```python
from build123d import *

# Parameters (mm, degrees)
F0_R     = 3.75
F0_R_2   = 1.75
F1_DEPTH = 3.8
F3_DEPTH = 2.5
F4_DEPTH = 1.2


with BuildPart() as f1:
    # F0 (on Top) → F1 (new body)
    with BuildSketch(Plane.XY):
        with Locations((56.9799989462, -33.0372825265)):
            Circle(F0_R)
        with Locations((56.9799989462, -33.0372825265)):
            Circle(F0_R_2, mode=Mode.SUBTRACT)
    extrude(amount=F1_DEPTH)

    # F2 (on face) → F3 (cut)
    with BuildSketch(Plane(origin=(0, 0, 0), x_dir=(1, 0, 0), z_dir=(0, 0, -1))):
        Polygon((59.8799989462, 31.3629667458), (59.8799989462, 34.7115983071), (56.9799989462, 36.3859140878), (54.0799989462, 34.7115983071), (54.0799989462, 31.3629667458), (56.9799989462, 29.6886509652), align=None)
    extrude(amount=-F3_DEPTH, mode=Mode.SUBTRACT)

    # F4 (add): a face of the model
    f4_faces = [f1.faces().sort_by_distance(p)[0] for p in [
        (53.3360649634, -33.0372825265, 3.8),
    ]]
    extrude(f4_faces, amount=F4_DEPTH)


solid = f1.part
```
The model under review builds one solid part; all positions refer to its coordinate system, in mm. A direction names the side the tool comes from. Coordinates: 2 decimals unless noted, no trailing zeros. Write each loop counter-clockwise with the first axis right and the second up, starting at its lowest first coordinate (ties: lowest second). Pieces come first, ordered by that corner, then holes.
1) We need section B-B on x = 57.5. State the section outline as (y, z) points.
2) The part is to be moulded in two halves that separate along X. For faces 3 (the face through (58, -30, 0)), 4 (the face through (56.49, -29.32, 2.46)), 5 (the face through (59.88, -33, 1)), say which applies: pulls with the +X half, pulls with the -X half, needs draft (parallel to the pull), parting line crosses it, or undercut.
3) Machinability: for faces 1 (the face through (58, -35, 5)), 2 (the face through (55.7, -31.6, 2.5)), which of the approach directions +Z, -Z, +X, -X, +Y, -Y give a long, thin tool a straight path to every point of the face, cutting with its end or side? Answer none if there is none.
4) We need section A-A on y = -33.75. State the section outline as (x, z) points, then the cut area to 3 significant figures.
5) To check wall thickness, follow probe 1 along Y at (x, z) = (57, 3.75); probe 2 along Z at (x, y) = (56.5, -30.75); probe 3 along X at (y, z) = (-32.5, 1.8). State the ranges of each line that lie inside material, in increasing order.
6) Clearance check with flat-ended pins moving along their axes: pin 1 Ø3 at (x, y) = (56.98, -33.04) entering from -Z; pin 2 Ø3 at (y, z) = (-36, 2) entering from +X; pin 3 Ø1 at (x, y) = (58, -35) entering from -Z. State where each tip first meets the part, or that it passes through.
7) We need section C-C on z = 2.1. State the section outline as (x, y) points, then the cut area to 3 significant figures.
8) We need section D-D on y = -35.25. State the section outline as (x, z) points, then the cut area to 3 significant figures.
Answer list:
1. outline: (-36.75, 0) - (-36.09, 0) - (-36.09, 2.5) - (-34.71, 2.5) - (-34.71, 5) - (-36.75, 5) - close; (-31.37, 2.5) - (-29.99, 2.5) - (-29.99, 0) - (-29.32, 0) - (-29.32, 5) - (-31.37, 5) - close
2. face 3: needs draft
2. face 4: parting line crosses it
2. face 5: undercut
3. face 1: +Z, +X, -X, +Y, -Y
3. face 2: -Z
4. outline: (53.3, 0) - (54.08, 0) - (54.08, 2.5) - (55.38, 2.5) - (55.38, 5) - (53.3, 5) - close; (58.58, 2.5) - (59.88, 2.5) - (59.88, 0) - (60.66, 0) - (60.66, 5) - (58.58, 5) - close
4. area: 14.3 mm2
5. probe 1: y = -36.79 to -34.79, -31.29 to -29.29
5. probe 2: z = 2.5 to 5
5. probe 3: x = 53.27 to 54.08, 59.88 to 60.69
6. pin 1: passes through
6. pin 2: stops at x = 60.43
6. pin 3: stops at z = 2.5
7. outline: circle Ø7.5 at (56.98, -33.04); hole (54.08, -34.71) - (56.98, -36.39) - (59.88, -34.71) - (59.88, -31.36) - (56.98, -29.69) - (54.08, -31.36) - close
7. area: 15.0 mm2
8. outline: (53.95, 0) - (55.01, 0) - (55.01, 2.5) - (58.95, 2.5) - (58.95, 0) - (60.01, 0) - (60.01, 5) - (53.95, 5) - close
8. area: 20.4 mm2
